Geometry check sheet. Reference: the model listing, model coordinates, mm. Face numbers are marked on the shaded views. A direction names the side the tool comes from. Coordinates: 2 decimals unless noted, no trailing zeros. Write each loop counter-clockwise with the first axis right and the second up, starting at its lowest first coordinate (ties: lowest second). Pieces come first, ordered by that corner, then holes. Notation, with made-up numbers: (22, 22) -> (78, 22) arc R26 ccw to (78, 43) -> close; hole circle Ø3 at (-10, -13). An arc over 180 degrees is marked (long way). Answer in a Markdown table with one row per item. Add a question column.
1. Cross-section at D-D on x = 164. Record the cut outline in (y, z), and give its area (3 significant figures).
2. Cross-section at A-A on z = 7. Record the cut outline in (x, y).
3. Cross-section at B-B on y = 9. Record the cut outline in (x, z), and give its area (3 significant figures).
4. Scan lines: L1, parallel to X at y = 11, z = 0; L2, parallel to Z at x = 79, y = 7.25; L3, parallel to Z at x = 79, y = 9.5. Record each from-to range of solid material in increasing order. Write a range as from..to.
5. Set-up check for the marked faces 1, 2 and 3: record each of +Z, -Z, +X, -X, +Y, -Y from which the full face is reachable in a straight line by a thin tool's end or side.
6. Cross-section at C-C on x = 79. Record the cut outline in (y, z), and give its area (3 significant figures).
7. Depth check by flat-ended pin: P1, Ø4, axis at x = 140, y = 17, coming from the -Z side; P2, Ø2.5, axis at x = 79, z = -0.5, coming from the +Y side; P3, Ø3, axis at x = 195, z = 2, coming from the +Y side. Enter the tip coordinate at first touch or a pass-through.
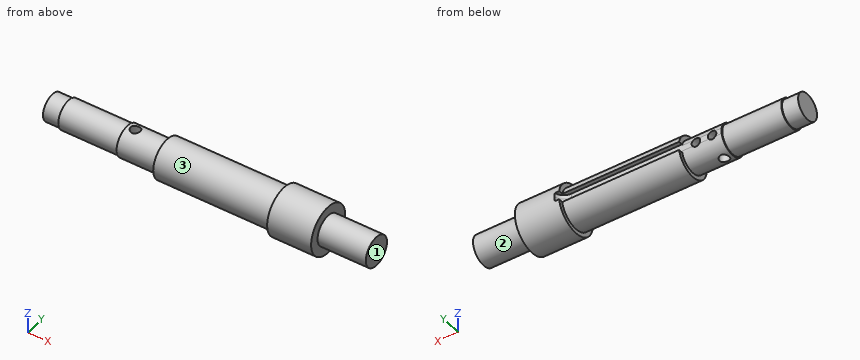
Autodesk Inventor part; units mm, degrees
ref_plane "Work Plane1" through (0, 17.5, 0) normal (0, 1, 0) x (-1, 0, 0)
ref_plane "Work Plane2" through (0, 14.25, 0) normal (0, 1, 0) x (-1, 0, 0)
ref_plane "Work Plane3" through (0, 0, -14.5) normal (0, 0, 1) x (1, 0, 0)
sketch "Sketch1" plane through (0, 0, 0) normal (0, 0, 1) x (1, 0, 0)
  line L0 (0, 0) -> (302, 0)
  line L1 (0, 0) -> (0, 12.5)
  line L2 (0, 12.5) -> (15, 12.5)
  line L3 (15, 12.5) -> (15, 13.5)
  line L4 (15, 13.5) -> (70, 13.5)
  line L5 (70, 13.5) -> (70, 14.5)
  line L6 (70, 14.5) -> (107, 14.5)
  line L7 (107, 14.5) -> (107, 18.5)
  line L8 (107, 18.5) -> (216, 18.5)
  line L9 (216, 18.5) -> (216, 22.5)
  line L10 (302, 0) -> (302, 14)
  line L11 (302, 14) -> (257, 14)
  line L12 (216, 22.5) -> (257, 22.5)
  line L13 (257, 22.5) -> (257, 14)
  dimension "d0" = 302
  dimension "d1" = 12.5
  dimension "d2" = 15
  dimension "d3" = 1
  dimension "d4" = 55
  dimension "d5" = 1
  dimension "d6" = 37
  dimension "d7" = 4
  dimension "d8" = 109
  dimension "d9" = 4
  dimension "d10" = 14
  dimension "d11" = 45
revolve "Revolution1" add sketch "Sketch1" angle 360 about axis through (0, 0, 0) along (1, 0, 0)
ref_plane "Work Plane1" through (0, 17.5, 0) normal (0, 1, 0) x (-1, 0, 0)
ref_plane "Work Plane2" through (0, 14.25, 0) normal (0, 1, 0) x (-1, 0, 0)
sketch "Sketch3" plane through (0, 14.25, 0) normal (0, 1, 0) x (-1, 0, 0)
  line L0 (-70, -4) -> (-220, -4)
  line L1 (-220, -4) -> (-220, 4)
  line L2 (-216, 22.5) -> (-216, -22.5)
  line L3 (-220, 4) -> (-70, 4)
  line L4 (-70, -4) -> (-70, 4)
  line L5 (-70, 14.5) -> (-70, -14.5)
  point P0 (0, 0)
  dimension "d17" = 150
  dimension "d18" = 8
  dimension "d19" = 150
extrude "Extrusion1" cut sketch "Sketch3" along normal blind 10
fillet "Fillet1" radius 10 1 edges at (220, 14.25, 0)
sketch "Sketch4" plane through (0, 14.25, 0) normal (0, 1, 0) x (1, 0, 0)
  circle A0 centre (79, 0) radius 4
  circle A1 centre (94, 0) radius 4
  line L0 (70, -2.681) -> (70, 2.681)
  point P0 (0, 0)
  dimension "d23" = 8
  dimension "d24" = 8
extrude "Extrusion2" cut sketch "Sketch4" against normal blind 9
ref_plane "Work Plane3" through (0, 0, -14.5) normal (0, 0, 1) x (1, 0, 0)
sketch "Sketch5" plane through (0, 0, -14.5) normal (0, 0, 1) x (1, 0, 0)
  circle A0 centre (77.4995, -0.0611) radius 4.5
  line L0 (70, -14.5) -> (70, 14.25)
  point P0 (0, 0)
  dimension "d31" = 9
extrude "Extrusion3" cut sketch "Sketch5" along normal blind 30
properties part number "eixo 2"
Results found:
| question | item | result |
|---|---|---|
| 1 | outline | (14.25, -4) -> (14.25, 4) -> (18.06, 4) arc R18.5 ccw (long way) to (18.06, -4) -> close |
| 1 | area | 1,040 mm^2 |
| 2 | outline | (0, -10.36) -> (15, -10.36) -> (15, -11.54) -> (70, -11.54) -> (70, -12.7) -> (107, -12.7) -> (107, -17.12) -> (216, -17.12) -> (216, -21.38) -> (257, -21.38) -> (257, -12.12) -> (302, -12.12) -> (302, 12.12) -> (257, 12.12) -> (257, 21.38) -> (216, 21.38) -> (216, 17.12) -> (107, 17.12) -> (107, 12.7) -> (70, 12.7) -> (70, 11.54) -> (15, 11.54) -> (15, 10.36) -> (0, 10.36) -> close; hole circle Ø9 at (77.5, -0.06) |
| 3 | outline | (0, -8.67) -> (15, -8.67) -> (15, -10.06) -> (70, -10.06) -> (70, -11.37) -> (107, -11.37) -> (107, -16.16) -> (216, -16.16) -> (216, -20.62) -> (257, -20.62) -> (257, -10.72) -> (302, -10.72) -> (302, 10.72) -> (257, 10.72) -> (257, 20.62) -> (216, 20.62) -> (216, 16.16) -> (107, 16.16) -> (107, 11.37) -> (70, 11.37) -> (70, 10.06) -> (15, 10.06) -> (15, 8.67) -> (0, 8.67) -> close; hole circle Ø8 at (79, 0); hole circle Ø8 at (94, 0) |
| 3 | area | 8,290 mm^2 |
| 4 | L1 | x = 0..75, 83..90, 98..302 |
| 4 | L2 | z = -12.56..-4, 4..12.56 |
| 4 | L3 | z = -10.95..-4, 4..10.95 |
| 5 | face 1 | +Z, -Z, +X, +Y, -Y |
| 5 | face 2 | +X |
| 5 | face 3 | -X |
| 6 | outline | (-4.3, -13.85) -> (-4.3, 13.85) arc R14.5 ccw to start; (4.18, -13.88) arc R14.5 ccw to (13.94, -4) -> (5.25, -4) -> (5.25, 4) -> (13.94, 4) arc R14.5 ccw to (4.18, 13.88) -> close |
| 6 | area | 346 mm^2 |
| 7 | P1 | stops at z = -10.83 |
| 7 | P2 | stops at y = 5.25 |
| 7 | P3 | stops at y = 14.25 |
